Input: dimensioned drawing with shaded views. Units: mm. Origin: part minimum x, y, z. A direction names the side the tool comes from. Round coordinates to 2 decimals unless told otherwise and drop trailing zeros. Order: outer loops, then holes, each group sorted by start corner. A loop starts at its lowest first (then second) coordinate and runs counter-clockwise, first axis right, second up.
Item 1: Cut plane A-A on z = 50.5. Output: boundary loops of the cut face in (x, y).
Item 2: Cut plane B-B on y = 111.5. Output: boundary loops of the cut face in (x, z).
Item 3: Mould query, pull axis X, two halves, no side actions, for the marked faces 1 and 2. Classes: released by +X, released by -X, zero draft, split by the parting line, or undercut.
Item 4: Reachability of the marked faces 3, 4, 5 and 6 from +Z, -Z, +X, -X, +Y, -Y: full face, straight path, thin tool, end or side. Return the list, or none.
Item 5: Cut plane C-C on x = 140.5. Output: boundary loops of the cut face in (y, z).
Item 6: Cut plane D-D on z = 120.5. Output: boundary loops of the cut face in (x, y).
Item 7: First-contact query: pin 1 (16 mm diameter, centred on y = 178, z = 8.5, fed in from -X); pin 2 (6 mm diameter, centred on x = 220.5, z = 110, fed in from -Y); pin 3 (17 mm diameter, centred on x = 139.5, y = 141, fed in from +Z). Flat tips, straight axial feed; report the tip coordinate or a pass-through.
Item 8: Line query: L1, parallel to X at y = 126.5, z = 8.5; L2, parallel to Z at x = 110, y = 204; L3, parallel to Y at x = 246.5, z = 127. Output: solid intervals per line, ascending.
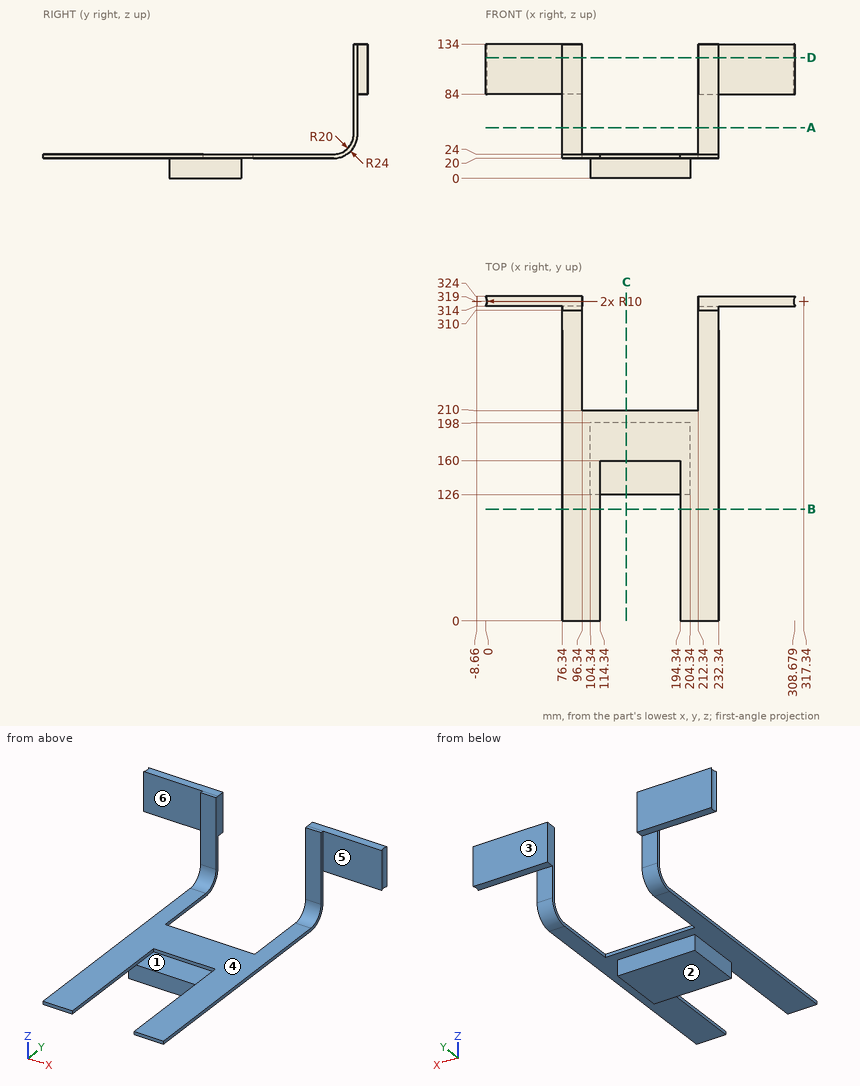
From the geometry:
1. outline: (76.34, 310) - (96.34, 310) - (96.34, 314) - (76.34, 314) - close; (212.34, 310) - (232.34, 310) - (232.34, 314) - (212.34, 314) - close
2. outline: (76.34, 20) - (114.34, 20) - (114.34, 24) - (76.34, 24) - close; (194.34, 20) - (232.34, 20) - (232.34, 24) - (194.34, 24) - close
3. face 1: undercut
3. face 2: zero draft
4. face 3: +Z, -Z, +X, -X, +Y
4. face 4: +Z, +X, -X, -Y
4. face 5: +Z, -Z, +X, -Y
4. face 6: +Z, -Z, -X, -Y
5. outline: (126, 0) - (198, 0) - (198, 20) - (210, 20) - (210, 24) - (160, 24) - (160, 20) - (126, 20) - close
6. outline: (0, 314) - (76.34, 314) - (76.34, 310) - (96.34, 310) - (96.34, 324) - (0, 324) arc R10 cw to start; (212.34, 310) - (232.34, 310) - (232.34, 314) - (308.68, 314) arc R10 cw to (308.68, 324) - (212.34, 324) - close
7. pin 1: stops at x = 104.34
7. pin 2: stops at y = 310
7. pin 3: stops at z = 20
8. L1: x = 104.34 to 204.34
8. L2: z = 20 to 24
8. L3: y = 314 to 324
